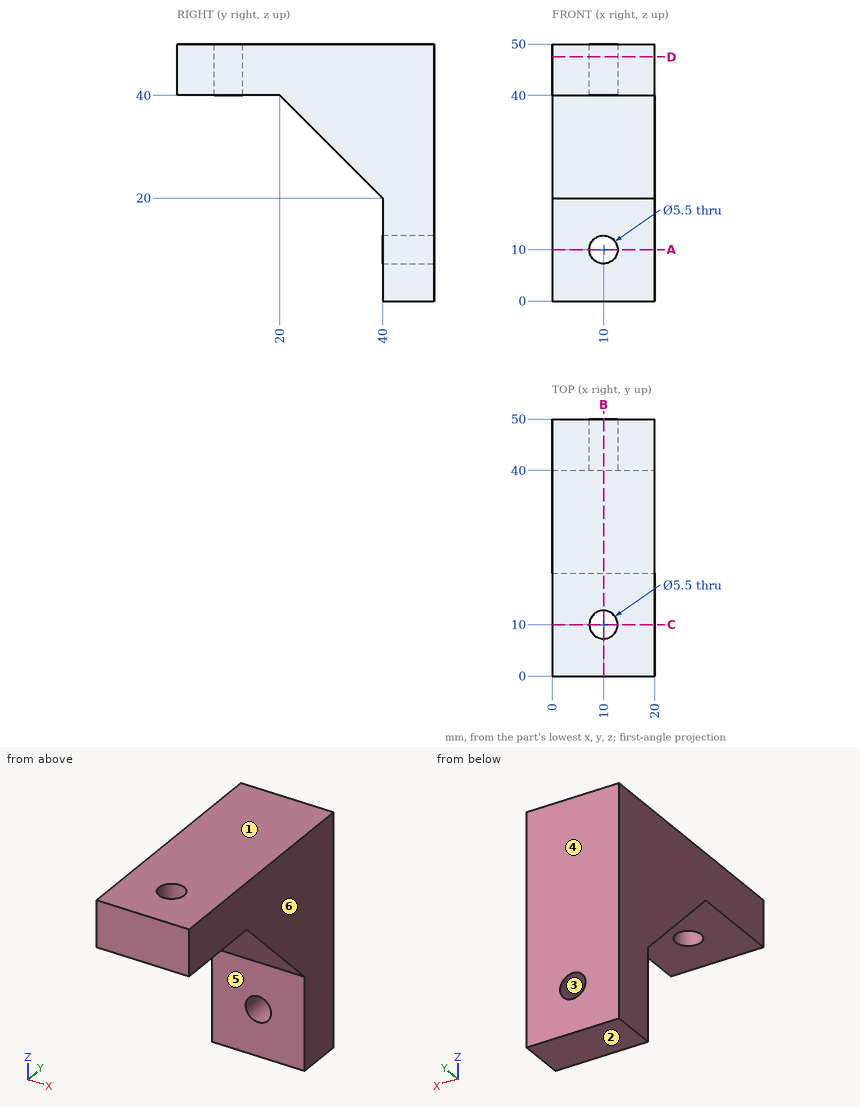
Drawing for the job (mm, zero at the part's lowest x, y, z). A direction names the side the tool comes from. Give positions to 0.01 mm unless a question says otherwise; leave off trailing zeros. Order: outer loops, then holes, each group sorted by start corner. A loop starts at its lowest first (then second) coordinate and runs counter-clockwise, first axis right, second up. Notation, with made-up numbers: M -37.5,63.5 L 11.5,63.5 A20 cw 11.5,88.5 Z; hole C 8,84 d9. An arc over 180 degrees is marked long. Use a Markdown table: item, result. Add a question column.
(1) Probe line 1 along X through (y, z) = (46, 10); line 2 along Z through (x, y) = (10, 46); line 3 along Y through (x, z) = (12.25, 2). List the from-to ranges inside material, lowest first. Write a range as [from, to].
(2) Mould opens along Z. For the marked faces 1, 2, 3 and 4 say: +Z half, -Z half, draft (parallel to the pull), parting line (faces both ways), or undercut.
(3) Saw through at B-B, the plane x = 10. Give the cut face in (y, z).
(4) Drop flat-ended pins along their axis: P1, Ø1, axis at x = 9.5, z = 26.5, coming from the -Y side; P2, Ø6, axis at x = 9.5, y = 32.5, coming from the -Z side; P3, Ø6.5, axis at x = 10, z = 10, coming from the -Y side; P4, Ø6, axis at x = 7, y = 44.5, coming from the -Z side. Give the stop position or say it passes through.
(5) Saw through at A-A, the plane z = 10. Give the cut face in (x, y).
(6) Saw through at D-D, the plane z = 47.5. Give the cut face in (x, y), and give its area (3 significant figures).
(7) 3-axis set-ups, long thin cutter, end or side, ignore diameter. For the marked faces 5 and 6: which of +Z, -Z, +X, -X, +Y, -Y reach the whole face in a straight line?
Answer key:
| question | item | result |
|---|---|---|
| 1 | line 1 | [0, 7.25], [12.75, 20] |
| 1 | line 2 | [0, 7.25], [12.75, 50] |
| 1 | line 3 | [40, 50] |
| 2 | face 1 | +Z half |
| 2 | face 2 | -Z half |
| 2 | face 3 | undercut |
| 2 | face 4 | draft |
| 3 | outline | M 0,40 L 7.25,40 L 7.25,50 L 0,50 Z; M 12.75,40 L 20,40 L 40,20 L 40,12.75 L 50,12.75 L 50,50 L 12.75,50 Z; M 40,0 L 50,0 L 50,7.25 L 40,7.25 Z |
| 4 | P1 | y = 33 |
| 4 | P2 | z = 24.5 |
| 4 | P3 | y = 40 |
| 4 | P4 | z = 0 |
| 5 | outline | M 0,40 L 7.25,40 L 7.25,50 L 0,50 Z; M 12.75,40 L 20,40 L 20,50 L 12.75,50 Z |
| 6 | outline | M 0,0 L 20,0 L 20,50 L 0,50 Z; hole C 10,10 d5.5 |
| 6 | area | 976 mm^2 |
| 7 | face 5 | -Z, +X, -X, -Y |
| 7 | face 6 | +Z, -Z, +X, +Y, -Y |
